from build123d import *

# Parameters (mm, degrees)
F0_W     = 30
F0_H     = 28
F0_R     = 4
F1_DEPTH = 18
F4_DEPTH = 40
F6_R     = 8
F7_R     = 8


# Not quite as in the source:
# - a fillet or chamfer that OpenCascade refuses, or shapes differently, is made with other operations: its cross-section is extruded or revolved along the edge and cut away or added


with BuildPart() as f1:
    # F0 (on Top) → F1 (new body)
    with BuildSketch(Plane.XY):
        with Locations((-30.3913680837, 12.4760417278)):
            Rectangle(F0_W, F0_H)
        with Locations((-30.3913680837, 4.4760417278)):
            Circle(F0_R, mode=Mode.SUBTRACT)
    extrude(amount=F1_DEPTH)

    # F2: chamfer of 2 x 8 on 1 edges, made by hand

    # F2_s1 → F2_t2 (revolve, cut)
    with BuildSketch(Plane.XZ.offset(-4.4760417278)):
        Polygon((-26.3913680837, 8), (-24.3913680837, 0), (-26.3913680837, 0), align=None)
    revolve(axis=Axis((-30.3913680837, 4.4760417278, 0), (0, 0, 1)), mode=Mode.SUBTRACT)

    # F3 (on face) → F4 (cut)
    with BuildSketch(Plane.YZ.offset(-15.3913680837)):
        with BuildLine():
            Line((18.4760417278, 10.8), (21.4760417278, 10.8))
            ThreePointArc((21.4760417278, 10.8), (23.5760417278, 12.9), (21.4760417278, 15))
            Line((21.4760417278, 15), (18.4760417278, 15))
            ThreePointArc((18.4760417278, 15), (16.3760417278, 12.9), (18.4760417278, 10.8))
        make_face()
    extrude(amount=-F4_DEPTH, mode=Mode.SUBTRACT)

    # F5: chamfer of 5 x 2 on 1 edges, made by hand

    # F5_s1 → F5_t2 (revolve, cut)
    with BuildSketch(Plane.XZ.offset(-4.4760417278)):
        Polygon((-24.3913680837, 18), (-26.3913680837, 13), (-26.3913680837, 18), align=None)
    revolve(axis=Axis((-30.3913680837, 4.4760417278, 18), (0, 0, 1)), mode=Mode.SUBTRACT)

    # F6
    f6_edges = [f1.edges().sort_by_distance(p)[0] for p in [
        (-34.391368, 4.476042, 13),
    ]]
    fillet(f6_edges, radius=F6_R)

    # F7
    f7_edges = [f1.edges().sort_by_distance(p)[0] for p in [
        (-34.391368, 4.476042, 8),
    ]]
    fillet(f7_edges, radius=F7_R)


solid = f1.part
Input: part model. Units: mm. Frame: model coordinates. A direction names the side the tool comes from. Give positions to 0.01 mm unless a question says otherwise; leave off trailing zeros. Order: outer loops, then holes, each group sorted by start corner. A loop starts at its lowest first (then second) coordinate and runs counter-clockwise, first axis right, second up. Notation, with made-up numbers: M 32.25,-7 L 42.25,-7 A36 cw 42.25,29 Z; hole C 6.25,49.25 d5. An arc over 180 degrees is marked long. Answer as a JSON object with one key per item and string values.
1. Cut plane D-D, the plane x = -32.25. State how many separate pieces and enclosed holes the cut face has, and give its area (3 significant figures).
Result sheet:
{"separate pieces": "2", "enclosed holes": "1", "area": "321 mm²"}
2. Ray query, line 1 (Y direction, x = -31.25, z = 12.5); line 2 (Z direction, x = -31.5, y = 19); line 3 (Y direction, x = -42.5, z = 11.75). Return the intervals inside material, ascending. Write a range as [from, to].
Result sheet:
{"line 1": "[-1.52, 0.5], [8.45, 16.41], [23.54, 26.48]", "line 2": "[0, 10.8], [15, 18]", "line 3": "[-1.52, 16.72], [23.23, 26.48]"}
3. Reachability of faces 5 (the flat face through (-31, -1.524, 9)), 6 (the flat face through (-30, 20, 15)) from +Z, -Z, +X, -X, +Y, -Y: full face, straight path, thin tool, end or side. Return the list, or none.
Result sheet:
{"face 5": "+Z, -Z, +X, -X, -Y", "face 6": "+X, -X"}
4. Pull-direction query (X, two-part tool) for faces 1 (the flat face through (-15.391, 12, 9)), 2 (the flat face through (-45.391, 12, 9)), 3 (the conical face through (-33.885, 7.68, 5.038)), 4 (the cylindrical face through (-30.181, 23.576, 12.854)); classes: +X half, -X half, draft (parallel to the pull), parting line (faces both ways), or undercut.
Result sheet:
{"face 1": "+X half", "face 2": "-X half", "face 3": "undercut", "face 4": "draft"}
5. Cut plane B-B, the plane y = 20.25. Output: boundary loops of the cut face in (x, z).
Result sheet:
{"outline": "M -45.39,0 L -15.39,0 L -15.39,10.8 L -45.39,10.8 Z; M -45.39,15 L -15.39,15 L -15.39,18 L -45.39,18 Z"}
6. First-contact query: P1, Ø5, axis at x = -30.39, y = 4.48, coming from the +Z side. Flat tip, straight axial feed; report the tip coordinate or a pass-through.
Result sheet:
{"P1": "through"}
7. Cut plane C-C, the plane z = 5.5. Output: boundary loops of the cut face in (x, y) (3 decimals).
Result sheet:
{"outline": "M -45.391,-1.524 L -15.391,-1.524 L -15.391,26.476 L -45.391,26.476 Z; hole C -30.391,4.476 d9.25"}
8. Cut plane A-A, the plane x = -37. Output: boundary loops of the cut face in (y, z), and give its area (3 significant figures).
Result sheet:
{"outline": "M -1.52,0 L 26.48,0 L 26.48,18 L -1.52,18 Z; hole M 18.48,10.8 L 21.48,10.8 A2.1 ccw 21.48,15 L 18.48,15 A2.1 ccw Z", "area": "478 mm²"}
